Check sheet for the drawn part. Datum: minimum x, y, z corner. Units: mm. A direction names the side the tool comes from. Give positions to 0.01 mm unless a question says otherwise; leave off trailing zeros. Loops run counter-clockwise (first coordinate to the right, second up) from the corner with the lowest first, then second, coordinate; pieces in that order, holes last. Notation, with made-up numbers: (16.5, 89) - (72.5, 89) arc R21 ccw to (72.5, 110) - close; hole circle Ø9 at (-35.75, -3). An arc over 180 degrees is marked (long way). Use a Markdown table: item, result. Add a question column.
1. Draft check along X on the marked faces 1, 2, 3 and 4. Enter one of: pulls with the +X half, pulls with the -X half, needs draft (parallel to the pull), parting line crosses it, or undercut.
2. Cross-section at B-B on z = 12.25. Enter the section's corners in (x, y), and give its area (3 significant figures).
3. Material ranges on L1, parallel to X at y = 12.75, z = 1.4; L2, parallel to Y at x = 1, z = 8.75; L3, parallel to Z at x = 1.75, y = 6.25, recorded low to high.
4. Cross-section at C-C on x = 9.11. Count the separate pieces of the cut face and the enclosed holes in it, and give its area (3 significant figures).
5. Cross-section at A-A on y = 12.75. Enter the section's corners in (x, z).
6. Set-up check for the marked faces 5 and 6: record each of +Z, -Z, +X, -X, +Y, -Y from which the full face is reachable in a straight line by a thin tool's end or side.
7. Depth check by flat-ended pin: P1, Ø6, axis at x = 5.5, y = 21, coming from the +Z side; P2, Ø1.5, axis at x = 9, z = 5, coming from the -Y side; P3, Ø1.5, axis at x = 4, y = 5.5, coming from the +Z side. Enter the tip coordinate at first touch or a pass-through.
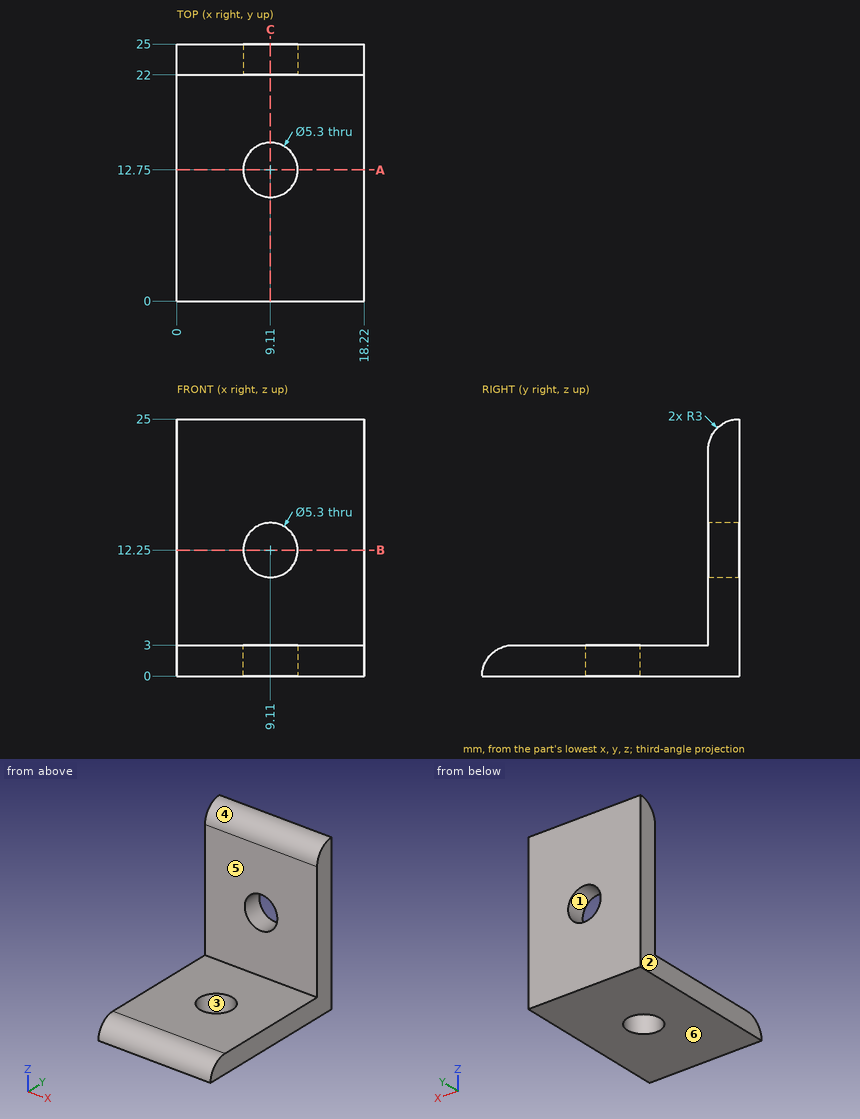
Values found:
| question | item | result |
|---|---|---|
| 1 | face 1 | undercut |
| 1 | face 2 | pulls with the -X half |
| 1 | face 3 | undercut |
| 1 | face 4 | needs draft |
| 2 | outline | (0, 22) - (6.46, 22) - (6.46, 25) - (0, 25) - close; (11.76, 22) - (18.22, 22) - (18.22, 25) - (11.76, 25) - close |
| 2 | area | 38.8 mm2 |
| 3 | L1 | x = 0 to 6.46, 11.76 to 18.22 |
| 3 | L2 | y = 22 to 25 |
| 3 | L3 | z = 0 to 3 |
| 4 | separate pieces | 3 |
| 4 | enclosed holes | 0 |
| 4 | area | 105 mm2 |
| 5 | outline | (0, 0) - (6.46, 0) - (6.46, 3) - (0, 3) - close; (11.76, 0) - (18.22, 0) - (18.22, 3) - (11.76, 3) - close |
| 6 | face 5 | +Z, +X, -X, -Y |
| 6 | face 6 | -Z, +X, -X, +Y, -Y |
| 7 | P1 | stops at z = 24.83 |
| 7 | P2 | stops at y = 22 |
| 7 | P3 | stops at z = 3 |
